Check sheet for the modelled part. Datum: model origin and axes. Units: mm. A direction names the side the tool comes from. Round coordinates to 2 decimals unless told otherwise and drop trailing zeros. Write each loop counter-clockwise with the first axis right and the second up, starting at its lowest first coordinate (ties: lowest second). Pieces come first, ordered by that corner, then holes.
from build123d import *

# Parameters (mm, degrees)
SKETCH1_R               = 2.25
BOSS_EXTRUDE1_DEPTH     = 5
SKETCH2_W               = 52.5
SKETCH2_H               = 52.5
SKETCH2_W_2             = 42.5
SKETCH2_H_2             = 42.5
BOSS_EXTRUDE2_DEPTH     = 40
BOSS_EXTRUDE3_DEPTH     = 36
CUT_EXTRUDE2_DEPTH      = 121.157448791
CUT_EXTRUDE2_DEPTH_BACK = 121.157448791
SKETCH6_R               = 2.5
CUT_EXTRUDE3_DEPTH      = 127.97834461
CUT_EXTRUDE3_DEPTH_BACK = 127.97834461
SKETCH7_R               = 2.5
SKETCH8_W               = 40
SKETCH8_H               = 36.5
CUT_EXTRUDE4_DEPTH      = 24
SKETCH9_W               = 25
SKETCH9_H               = 25.519409936
CUT_EXTRUDE5_DEPTH      = 2.35


with BuildPart() as part:
    # Sketch1 → Boss-Extrude1 (new body)
    with BuildSketch(Plane.XY):
        Polygon((0, 30), (-9.25, 30), (-9.25, 82.5), (43.25, 82.5), (43.25, 30), (34, 30), (34, 0), (0, 0), align=None)
        with Locations((4.75, 25.25)):
            Circle(SKETCH1_R, mode=Mode.SUBTRACT)
        with Locations((29.25, 25.25)):
            Circle(SKETCH1_R, mode=Mode.SUBTRACT)
        with Locations((29.25, 4.75)):
            Circle(SKETCH1_R, mode=Mode.SUBTRACT)
        with Locations((4.75, 4.75)):
            Circle(SKETCH1_R, mode=Mode.SUBTRACT)
    extrude(amount=BOSS_EXTRUDE1_DEPTH)

    # Sketch2 → Boss-Extrude2 (add)
    with BuildSketch(Plane.XY.offset(5)):
        with Locations((17, 56.25)):
            Rectangle(SKETCH2_W, SKETCH2_H)
        with Locations((17, 56.25)):
            Rectangle(SKETCH2_W_2, SKETCH2_H_2, mode=Mode.SUBTRACT)
    extrude(amount=BOSS_EXTRUDE2_DEPTH)

    # Sketch5 → Boss-Extrude3 (add)
    with BuildSketch(Plane.XY.offset(45)):
        Polygon((43.25, 82.5), (43.25, 30), (13.25, 30), (13.25, 35), (38.25, 35), (38.25, 77.5), (13.25, 77.5), (13.25, 82.5), align=None)
    extrude(amount=BOSS_EXTRUDE3_DEPTH)

    # Sketch6 → Cut-Extrude2 (cut, two sides: drawn at the far end of the back side and taken through both)
    with BuildSketch(Plane.XZ.offset(-77.5).offset(-CUT_EXTRUDE2_DEPTH_BACK)):
        with Locations(Location((20.75, 73.5, 0), (0, 0, 270))):
            Circle(SKETCH6_R)
    extrude(amount=CUT_EXTRUDE2_DEPTH + CUT_EXTRUDE2_DEPTH_BACK, mode=Mode.SUBTRACT)

    # Sketch7 → Cut-Extrude3 (cut, two sides: drawn at the far end of the back side and taken through both)
    with BuildSketch(Plane(origin=(43.25, 0, 0), x_dir=(0, 0, -1), z_dir=(1, 0, 0)).offset(-CUT_EXTRUDE3_DEPTH_BACK)):
        with Locations(Location((-71, 55.075, 0), (0, 0, 90))):
            Circle(SKETCH7_R)
    extrude(amount=CUT_EXTRUDE3_DEPTH + CUT_EXTRUDE3_DEPTH_BACK, mode=Mode.SUBTRACT)

    # Sketch8 → Cut-Extrude4 (cut)
    with BuildSketch(Plane.ZY.offset(9.25)):
        with Locations((25, 56.25)):
            Rectangle(SKETCH8_W, SKETCH8_H)
    extrude(amount=-CUT_EXTRUDE4_DEPTH, mode=Mode.SUBTRACT)

    # Sketch9 → Cut-Extrude5 (cut)
    with BuildSketch(Plane(origin=(0, 35, 0), x_dir=(1, 0, 0), z_dir=(0, 1, 0))):
        with Locations((25.75, -68.240295032)):
            Rectangle(SKETCH9_W, SKETCH9_H)
    extrude(amount=-CUT_EXTRUDE5_DEPTH, mode=Mode.SUBTRACT)


solid = part.part
1. Sectioned sample at C-C, the plane z = 48. Enter the section's corners in (x, y).
2. Release check for a two-part mould opening along Z. For faces 1 (the cylindrical face through (40.715, 52.577, 71.11)), 2 (the flat face through (39, 62, 81)), 3 (the flat face through (17, 51, 0)), 4 (the flat face through (-7, 38, 25)) record: released by +Z, released by -Z, zero draft, split by the parting line, or undercut.
3. Scan lines: line 1 along Y through (x, z) = (4.75, 3.1); line 2 along Y through (x, z) = (28.5, 7); line 3 along X through (y, z) = (81.15, 73.5). Record each from-to range of solid material in increasing order.
4. Set-up check for faces 5 (the flat face through (26, 34, 55.481)), 6 (the flat face through (17, 15, 5)), 7 (the flat face through (34, 15, 2)), 8 (the flat face through (2, 79, 45)), 9 (the flat face through (17, 35, 30)): record each of +Z, -Z, +X, -X, +Y, -Y from which the full face is reachable in a straight line by a thin tool's end or side.
5. Go/stop test with flat-tipped pins: pin 1 (1.5 mm diameter, centred on x = -8, z = 33.5, fed in from -Y); pin 2 (10 mm diameter, centred on y = 9, z = 10.5, fed in from -X); pin 3 (1.2 mm diameter, centred on x = 31, y = 34, fed in from +Z); pin 4 (5 mm diameter, centred on x = 29.25, y = 4.75, fed in from -Z). Record where each tip stops, or that it passes through.
6. Sectioned sample at B-B, the plane y = 25.25. Enter the section's corners in (x, z).
7. Sectioned sample at D-D, the plane x = 20.75. Enter the section's corners in (y, z), plus the area to 3 significant figures.
8. Sectioned sample at A-A, the plane x = 4.75. Enter the section's corners in (y, z), plus the area to 4 significant figures.
Computed values:
1. outline: (13.25, 30) - (43.25, 30) - (43.25, 82.5) - (13.25, 82.5) - (13.25, 77.5) - (38.25, 77.5) - (38.25, 35) - (13.25, 35) - close
2. face 1: undercut
2. face 2: released by +Z
2. face 3: released by -Z
2. face 4: zero draft
3. line 1: y = 0 to 2.5, 7 to 23, 27.5 to 82.5
3. line 2: y = 30 to 35, 77.5 to 82.5
3. line 3: x = 13.25 to 18.25, 23.25 to 43.25
4. face 5: +Z, -X
4. face 6: +Z, +X, -X, -Y
4. face 7: +Z, -Z, +X, -Y
4. face 8: +Z, -X, +Y, -Y
4. face 9: +Z
5. pin 1: stops at y = 30
5. pin 2: passes through
5. pin 3: stops at z = 55.48
5. pin 4: stops at z = 0
6. outline: (0, 0) - (2.5, 0) - (2.5, 5) - (0, 5) - close; (7, 0) - (27, 0) - (27, 5) - (7, 5) - close; (31.5, 0) - (34, 0) - (34, 5) - (31.5, 5) - close
7. outline: (0, 0) - (82.5, 0) - (82.5, 71) - (77.5, 71) - (77.5, 5) - (35, 5) - (35, 55.48) - (32.65, 55.48) - (32.65, 71) - (30, 71) - (30, 5) - (0, 5) - close; (30, 76) - (32.65, 76) - (32.65, 81) - (30, 81) - close; (77.5, 76) - (82.5, 76) - (82.5, 81) - (77.5, 81) - close
7. area: 1,070 mm2
8. outline: (0, 0) - (2.5, 0) - (2.5, 5) - (0, 5) - close; (7, 0) - (23, 0) - (23, 5) - (7, 5) - close; (27.5, 0) - (82.5, 0) - (82.5, 45) - (77.5, 45) - (77.5, 5) - (35, 5) - (35, 45) - (30, 45) - (30, 5) - (27.5, 5) - close
8. area: 767.5 mm2
